The listing builds one solid part. Answer for the finished solid, in the listing's coordinates (mm). A direction names the side the tool comes from. Coordinates: 2 decimals unless noted, no trailing zeros. Loops run counter-clockwise (first coordinate to the right, second up) from the corner with the lowest first, then second, coordinate; pieces in that order, holes last. Notation, with made-up numbers: (-11.75, -39) - (21.25, -39) arc R25 cw to (21.25, -12) - close; hole circle Ø7 at (83, -12.75). An arc over 180 degrees is marked (long way). One line per question, with ' | ' between items.
from build123d import *

# Parameters (mm, degrees)
BOSS_EXTRUDE1_DEPTH = 20
FILLET1_R           = 10
CUT_EXTRUDE1_REACH  = 94.331
SKETCH4_R           = 5
SKETCH5_R           = 10
BOSS_EXTRUDE2_DEPTH = 20


with BuildPart() as part:
    # Sketch1 → Boss-Extrude1 (new body)
    with BuildSketch(Plane.XY):
        with BuildLine():
            Line((0, 15), (85, 15))
            Line((85, 15), (85, -5))
            Line((85, -5), (65, -5))
            Line((65, -5), (65, -15))
            Line((65, -15), (0, -15))
            ThreePointArc((0, -15), (-15, 0), (0, 15))
        make_face()
    extrude(amount=-BOSS_EXTRUDE1_DEPTH)

    # Fillet1
    fillet1_edges = [part.edges().sort_by_distance(p)[0] for p in [
        (85, 5, 0),
        (85, 5, -20),
    ]]
    fillet(fillet1_edges, radius=FILLET1_R - 0.0001)  # a hair under: the kernel refuses the full size

    # Sketch4 → Cut-Extrude1 (cut, up to next)
    with BuildSketch(Plane(origin=(0, 15, 0), x_dir=(1, 0, 0), z_dir=(0, 1, 0)), mode=Mode.PRIVATE) as cut_extrude1_sk1:
        with Locations(Location((75, 10, 0), (0, 0, 270))):
            Circle(SKETCH4_R)
    cut_extrude1_tool1 = extrude(cut_extrude1_sk1.sketch, amount=-CUT_EXTRUDE1_REACH, mode=Mode.PRIVATE) & part.part
    add(cut_extrude1_tool1.solids().sort_by_distance((75, 15, -10))[0], mode=Mode.SUBTRACT)

    # Sketch5 → Boss-Extrude2 (add)
    with BuildSketch(Plane(origin=(0, 0, -20), x_dir=(-1, 0, 0), z_dir=(0, 0, -1))):
        with Locations(Location((0, 0, 0), (0, 0, 180))):
            Circle(SKETCH5_R)
    extrude(amount=BOSS_EXTRUDE2_DEPTH)


solid = part.part
Item 1: Find section B-B, the plane x = 76. Write down the section's boundary in (y, z).
Taken from the geometry:
outline: (-5, -19.95) - (15, -19.95) - (15, -14.9) - (-5, -14.9) - close; (-5, -5.1) - (15, -5.1) - (15, -0.05) - (-5, -0.05) - close
Item 2: Find section D-D, the plane y = -7. Write down the section's boundary in (x, z).
Taken from the geometry:
outline: (-13.27, -20) - (-7.14, -20) - (-7.14, -40) - (7.14, -40) - (7.14, -20) - (65, -20) - (65, 0) - (-13.27, 0) - close
Item 3: Which of the six approach directions +Z, -Z, +X, -X, +Y, -Y give full straight-line access (tool end or side, diameter ignored) to faces 4 (the face through (42, 15, -10)), 5 (the face through (65, -10, -10))?
Taken from the geometry:
face 4: +Z, -Z, +X, -X, +Y | face 5: +Z, -Z, +X, -Y
Item 4: Each of these flat-tipped pins is pushed along its axis until it touches: pin 1 Ø4 at (y, z) = (-8, -36) entering from -X; pin 2 Ø5 at (y, z) = (-8.5, -5.5) entering from +X; pin 3 Ø3 at (y, z) = (-2, -30) entering from +X; pin 4 Ø6 at (x, z) = (75, -10) entering from +Y. Where does it stop, or does it pass through?
Taken from the geometry:
pin 1: stops at x = -8 | pin 2: stops at x = 65 | pin 3: stops at x = 9.99 | pin 4: passes through
Item 5: The mould has two halves that part along Z. Classify faces 1 (the face through (82.15, 4.86, -3.01)), 2 (the face through (-10, 0, -30)), 3 (the face through (70.12, 5.14, -11.08)): pulls with the +Z half, pulls with the -Z half, needs draft (parallel to the pull), parting line crosses it, or undercut.
Taken from the geometry:
face 1: pulls with the +Z half | face 2: needs draft | face 3: undercut
Item 6: Find section C-C, the plane z = -36. Write down the section's boundary in (x, y), plus the area to 3 significant figures.
Taken from the geometry:
outline: circle Ø20 at (0, 0) | area: 314 mm2
Item 7: Find the intervals of material crossed by line 1 (Z direction, x = 28, y = 2); line 2 (Y direction, x = 69.5, z = -16); line 3 (X direction, y = 8.5, z = -10), in increasing order. Write a range as [from, to].
Taken from the geometry:
line 1: z = [-20, 0] | line 2: y = [-5, 15] | line 3: x = [-12.36, 70], [80, 85]
